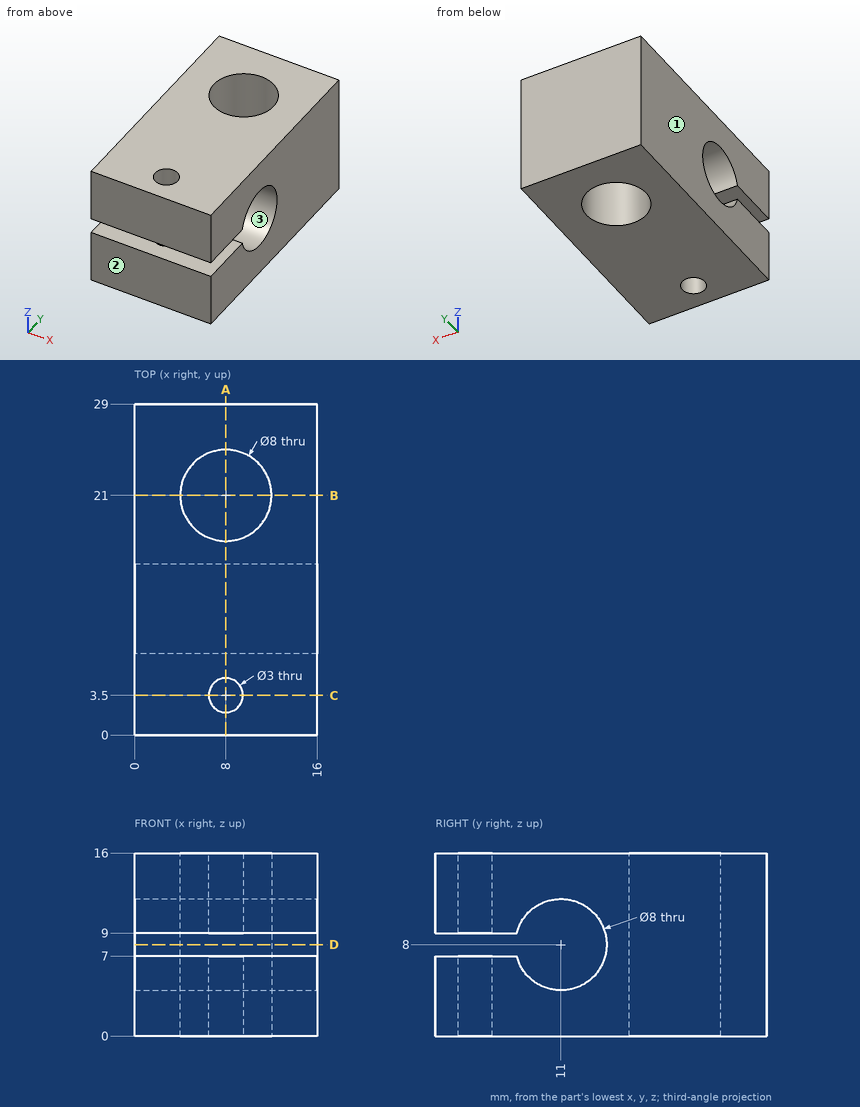
Could you check a few things on this drawing? It's one solid part, dimensions in mm from its lowest x, y, z. Coordinates: 2 decimals unless noted, no trailing zeros. Order: outer loops, then holes, each group sorted by start corner. A loop starts at its lowest first (then second) coordinate and runs counter-clockwise, first axis right, second up.
1) I need wall thicknesses on line 1 (Y direction, x = 8, z = 12.5); line 2 (Z direction, x = 11, y = 5); line 3 (Y direction, x = 8, z = 11.25). Which ranges of each line are inside material? Lowest first, please.
2) Will these pins go through, and if not, where does the flat tip stop? pin 1 (3.5 mm diameter, centred on x = 8, y = 4.5, fed in from -Z); pin 2 (2.5 mm diameter, centred on x = 8, y = 3.5, fed in from +Z).
3) Imagine slicing it at A-A on x = 8. List the corners of the cut face in (y, z) for me.
4) Imagine slicing it at C-C on y = 3.5. List the corners of the cut face in (x, z) for me, and give its area (3 significant figures).
5) Imagine slicing it at D-D on z = 8. List the corners of the cut face in (x, y) for me, and give its area (3 significant figures).
6) We'd pull the mould along Y, two halves only. Please class the marked faces 1, 2 and 3: +Y half, -Y half, draft (parallel to the pull), parting line (faces both ways), or undercut.
7) Imagine slicing it at B-B on y = 21. List the corners of the cut face in (x, z) for me, and give its area (3 significant figures).
Response values:
1. line 1: y = 0 to 2, 5 to 17, 25 to 29
1. line 2: z = 0 to 7, 9 to 16
1. line 3: y = 0 to 2, 5 to 8.67, 13.33 to 17, 25 to 29
2. pin 1: stops at z = 0
2. pin 2: passes through
3. outline: (0, 0) - (2, 0) - (2, 7) - (0, 7) - close; (0, 9) - (2, 9) - (2, 16) - (0, 16) - close; (5, 0) - (17, 0) - (17, 16) - (5, 16) - (5, 9) - (7.13, 9) arc R4 cw (long way) to (7.13, 7) - (5, 7) - close; (25, 0) - (29, 0) - (29, 16) - (25, 16) - close
4. outline: (0, 0) - (6.5, 0) - (6.5, 7) - (0, 7) - close; (0, 9) - (6.5, 9) - (6.5, 16) - (0, 16) - close; (9.5, 0) - (16, 0) - (16, 7) - (9.5, 7) - close; (9.5, 9) - (16, 9) - (16, 16) - (9.5, 16) - close
4. area: 182 mm2
5. outline: (0, 15) - (16, 15) - (16, 29) - (0, 29) - close; hole circle Ø8 at (8, 21)
5. area: 174 mm2
6. face 1: draft
6. face 2: -Y half
6. face 3: undercut
7. outline: (0, 0) - (4, 0) - (4, 16) - (0, 16) - close; (12, 0) - (16, 0) - (16, 16) - (12, 16) - close
7. area: 128 mm2
